Part model, mm, in its own coordinate system. A direction names the side the tool comes from. Coordinates: 2 decimals unless noted, no trailing zeros. Write each loop counter-clockwise with the first axis right and the second up, starting at its lowest first coordinate (ties: lowest second). Pieces come first, ordered by that corner, then holes. Notation, with made-up numbers: (51, 49.25) -> (64, 49.25) arc R23 cw to (64, 71.25) -> close; hole circle Ø7 at (-9.75, 19.5). An arc over 180 degrees is marked (long way). Write item = value, one per line.
from build123d import *

# Parameters (mm, degrees)
CUT_EXTRUDE1_START = 11.6078
CUT_EXTRUDE1_DEPTH = 2.0828


with BuildPart() as part:
    # Sketch2 → Revolve1 (revolve)
    with BuildSketch(Plane(origin=(0, 0, 0), x_dir=(0, 0, -1), z_dir=(1, 0, 0)), mode=Mode.PRIVATE) as revolve1_sk:
        with BuildLine():
            Line((11.6078, 0), (11.6078, 1.60655))
            Line((11.6078, 1.60655), (11.13155, 2.0828))
            Line((11.13155, 2.0828), (-7.4422, 2.0828))
            Line((-7.4422, 2.0828), (-7.4422, 3.22072))
            ThreePointArc((-7.4422, 3.22072), (-7.5032038, 3.3679962), (-7.65048, 3.429))
            Line((-7.65048, 3.429), (-11.39952, 3.429))
            ThreePointArc((-11.39952, 3.429), (-11.5467962, 3.3679962), (-11.6078, 3.22072))
            Line((-11.6078, 3.22072), (-11.6078, 0))
            Line((-11.6078, 0), (11.6078, 0))
        make_face()
    revolve(revolve1_sk.sketch.rotate(Axis((0, 0, -11.6078), (0, 0, 1)), 90), axis=Axis((0, 0, -11.6078), (0, 0, 1)))

    # Sketch3 → Cut-Extrude1 (cut)
    with BuildSketch(Plane.XY.offset(CUT_EXTRUDE1_START)):
        Polygon((-1.7859375, 1.031111496), (-1.7859375, -1.031111496), (0, -2.062222993), (1.7859375, -1.031111496), (1.7859375, 1.031111496), (0, 2.062222993), align=None)
    extrude(amount=-CUT_EXTRUDE1_DEPTH, mode=Mode.SUBTRACT)

    # Cut-Extrude2 cone 1 section (through the dimple's axis) → Cut-Extrude2 (revolve, cut)
    with BuildSketch(Plane(origin=(0, 0, 11.6078), x_dir=(0, -1, 0), z_dir=(1, 0, 0))):
        Polygon((0, 0), (2.255305827, 0), (0, 1.302101426), align=None)
    revolve(axis=Axis((0, 0, 11.6078), (0, 0, -1)), mode=Mode.SUBTRACT)


solid = part.part
Q1. Pin check, flat tips, straight feed: pin 1 (2 mm diameter, centred on y = -2.5, z = -1, fed in from +X) (3 decimals); pin 2 (1 mm diameter, centred on x = -2.5, y = 2, fed in from -Z); pin 3 (1.5 mm diameter, centred on x = 0, z = -9, fed in from +Y). Stop position of each tip, or through.
Model answer:
pin_1 = 1.445
pin_2 = 7.44
pin_3 = 2.08
Q2. Which spindle directions (+Z, -Z, +X, -X, +Y, -Y) get a long thin tool onto all of the face, cutting with end or side? Do faces 5 (the face through (2, 1, 7.442)), 6 (the face through (0.74, 3.35, 9.55)), 7 (the face through (0, 0, 9.525)). Say none if no direction does.
Model answer:
face_5 = -Z
face_6 = +Z, -Z
face_7 = +Z
Q3. Saw through at B-B on z = 6.75. Give the cut face in (x, y).
Model answer:
outline = circle Ø4.17 at (0, 0)
Q4. Probe line 1 (Z direction, x = -1.25, y = -2); line 2 (X direction, y = -0.25, z = 6.75); line 3 (Z direction, x = 1, y = 0.25) (3 decimals). List the from-to ranges inside material, lowest first. Write a range as from..to.
Model answer:
line_1 = 7.44..11.61
line_2 = -2.07..2.07
line_3 = -11.608..9.525
Q5. Mould opens along Y. For faces 1 (the face through (-1.987, -0.626, -1.715)), 2 (the face through (0.88, -1.554, 10.524)), 3 (the face through (0.905, 1.539, 10.524)), 4 (the face through (-1.4, 2.1, 11.608)) say: released by +Y, released by -Y, zero draft, split by the parting line, or undercut.
Model answer:
face_1 = split by the parting line
face_2 = undercut
face_3 = undercut
face_4 = zero draft
Q6. Saw through at A-A on y = 0. Give the cut face in (x, z) (3 decimals).
Model answer:
outline = (-3.429, 7.65) arc R0.208 ccw to (-3.221, 7.442) -> (-2.083, 7.442) -> (-2.083, -11.132) -> (-1.607, -11.608) -> (1.607, -11.608) -> (2.083, -11.132) -> (2.083, 7.442) -> (3.221, 7.442) arc R0.208 ccw to (3.429, 7.65) -> (3.429, 11.4) arc R0.208 ccw to (3.221, 11.608) -> (2.255, 11.608) -> (1.786, 11.337) -> (1.786, 9.525) -> (-1.786, 9.525) -> (-1.786, 11.337) -> (-2.255, 11.608) -> (-3.221, 11.608) arc R0.208 ccw to (-3.429, 11.4) -> close
